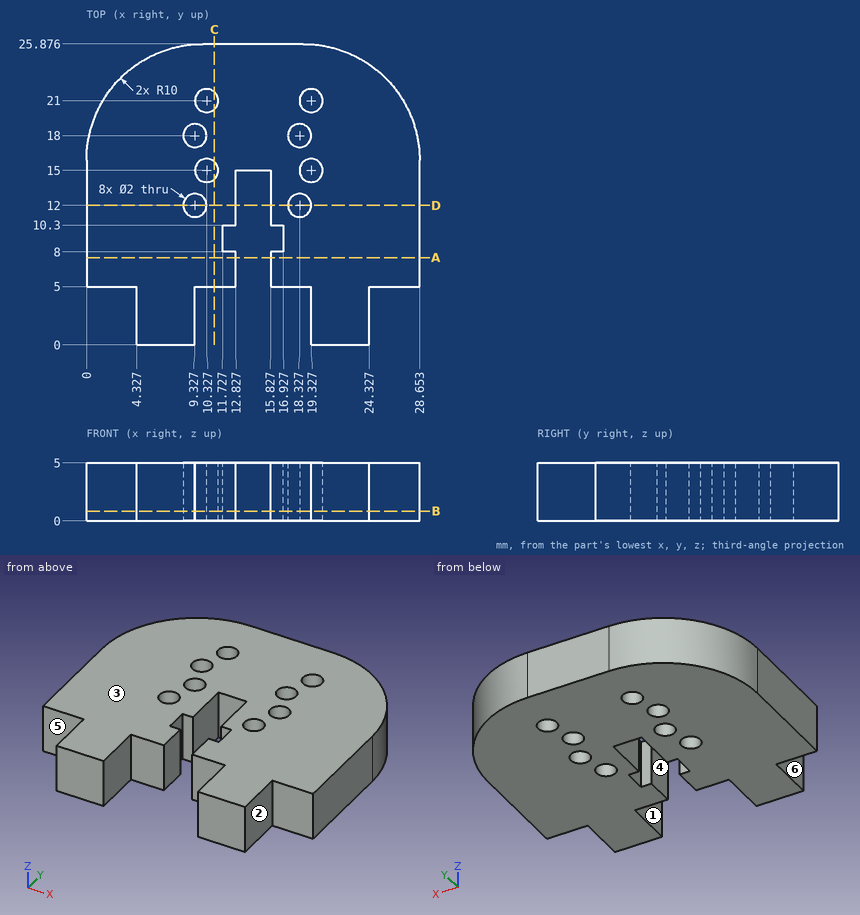
Geometry: see drawing. Coordinates: mm, zero at the bounding-box minimum. A direction names the side the tool comes from. Round coordinates to 2 decimals unless told otherwise and drop trailing zeros. Order: outer loops, then holes, each group sorted by start corner. A loop starts at its lowest first (then second) coordinate and runs counter-clockwise, first axis right, second up. Notation, with made-up numbers: (29, -24.75) - (46, -24.75) arc R27 cw to (46, 12.25) - close; hole circle Ø11 at (-18, -4.5). An arc over 180 degrees is marked (long way). One line per question, with ' | ' between items. Start each with the question number.
1) Cut plane D-D, the plane y = 12. Return the cut outline in (x, z).
2) Contact query for flat-ended pins moving along their axis: P1, Ø1.2, axis at x = 16, z = 2, coming from the -Y side; P2, Ø1.5, axis at y = 2.5, z = 3, coming from the +X side; P3, Ø1.5, axis at y = 2, z = 2.5, coming from the -X side. Output: stop coordinate, or through.
3) Cut plane C-C, the plane x = 11. Return the cut outline in (y, z).
4) Cut plane A-A, the plane y = 7.5. Return the cut outline in (x, z), then the cut area to 3 significant figures.
5) Pull-direction query (X, two-part tool) for the marked faces 4, 5 and 6; classes: +X half, -X half, draft (parallel to the pull), parting line (faces both ways), or undercut.
6) Set-up query: the marked faces 1, 2 and 3. Return all of +Z, -Z, +X, -X, +Y, -Y with unobstructed straight access to the full face (end or side cutting, diameter ignored); none if empty.
7) Cut plane B-B, the plane z = 0.85. Give the number of separate pieces and of enclosed holes in the cut face, then the cut area to 3 significant figures.
8) Ray query, probe 1 along X at (y, z) = (13.75, 3.95); probe 2 along Y at (x, z) = (19.75, 2.9) (1 decimal); probe 3 along Y at (x, z) = (16.5, 2.15). Return the intervals inside material, ascending.
Worked out:
1) outline: (0, 0) - (8.33, 0) - (8.33, 5) - (0, 5) - close; (10.33, 0) - (12.83, 0) - (12.83, 5) - (10.33, 5) - close; (15.83, 0) - (17.33, 0) - (17.33, 5) - (15.83, 5) - close; (19.33, 0) - (28.65, 0) - (28.65, 5) - (19.33, 5) - close
2) P1: stops at y = 5 | P2: stops at x = 24.33 | P3: stops at x = 4.33
3) outline: (5, 0) - (14.26, 0) - (14.26, 5) - (5, 5) - close; (15.74, 0) - (20.26, 0) - (20.26, 5) - (15.74, 5) - close; (21.74, 0) - (25.88, 0) - (25.88, 5) - (21.74, 5) - close
4) outline: (0, 0) - (12.83, 0) - (12.83, 5) - (0, 5) - close; (15.83, 0) - (28.65, 0) - (28.65, 5) - (15.83, 5) - close | area: 128 mm^2
5) face 4: undercut | face 5: draft | face 6: -X half
6) face 1: +Z, -Z, -Y | face 2: +Z, -Z, +X, -Y | face 3: +Z, +X, -X, +Y, -Y
7) separate pieces: 1 | enclosed holes: 8 | area: 545 mm^2
8) probe 1: x = 0 to 12.83, 15.83 to 28.65 | probe 2: y = 0 to 14.1, 15.9 to 20.1, 21.9 to 25.8 | probe 3: y = 5 to 8, 10.3 to 25.88
